Autodesk Inventor part; units mm, degrees
ref_plane "YZ Plane" through (0, 0, 0) normal (1, 0, 0) x (0, 1, 0)
ref_plane "XZ Plane" through (0, 0, 0) normal (0, 1, 0) x (-1, 0, 0)
ref_plane "XY Plane" through (0, 0, 0) normal (0, 0, 1) x (1, 0, 0)
sketch "Sketch1" plane through (0, 0, 0) normal (1, 0, 0) x (0, 1, 0)
  circle A0 centre (0, 0) radius 15.875
  circle A1 centre (18.7452, -32.4676) radius 4.0043
  circle A2 centre (18.7452, -32.4676) radius 15.875
  circle A3 centre (-37.4904, 0) radius 4.0043
  circle A4 centre (-37.4904, 0) radius 15.875
  circle A5 centre (18.7452, 32.4676) radius 15.875
  circle A6 centre (18.7452, 32.4676) radius 4.0043
  circle A7 centre (18.7452, -32.4676) radius 4.0043
  circle A8 centre (18.7452, -32.4676) radius 15.875
  circle A9 centre (0, 0) radius 15.875
  circle A10 centre (-37.4904, 0) radius 4.0043
  circle A11 centre (-37.4904, 0) radius 15.875
  circle A12 centre (18.7452, 32.4676) radius 4.0043
  circle A13 centre (18.7452, 32.4676) radius 15.875
  line L0 (34.6202, 32.4676) -> (34.6202, -32.4676)
  line L1 (10.8077, -46.2158) -> (-45.4279, -13.7482)
  line L2 (10.8077, 46.2158) -> (-45.4279, 13.7482)
  circle A14 centre (18.7452, 32.4676) radius 15.875
  circle A15 centre (-37.4904, 0) radius 15.875
  circle A16 centre (18.7452, -32.4676) radius 15.875
  circle A17 centre (41.995, 0) radius 14.4142
  circle A18 centre (-20.9975, 36.3687) radius 14.4142
  circle A19 centre (-20.9975, -36.3687) radius 14.4142
  point P0 (-28.0356, -23.7896)
  point P1 (-6.5846, -36.1743)
  point P2 (10.8077, -46.2158)
  point P3 (34.6202, -12.3847)
  point P4 (34.6202, 12.3847)
  point P5 (-6.5846, 36.1743)
  point P6 (-28.0356, 23.7896)
  point P7 (-45.4279, 13.7482)
  point P8 (-45.4279, -13.7482)
  dimension "d28" = 360
  dimension "d34" = 31.75
  dimension "d35" = 28.8284
  dimension "d36" = 8.0086
  dimension "d37" = 31.75
  dimension "d38" = 31.75
  dimension "d39" = 60
  dimension "d40" = 60
  dimension "d41" = 7.3748
  dimension "d42" = 55.6177
  dimension "d43" = 55.6177
  dimension "d44" = 0
  dimension "d45" = 41.2048
  dimension "d46" = 0
  dimension "d47" = 62.6558
  dimension "d48" = 80.0481
  dimension "d49" = 0
  dimension "d50" = 80.0481
  dimension "d51" = 15.875
  dimension "d52" = 15.875
  dimension "d53" = 23.8125
  dimension "d54" = 80.0481
  dimension "d55" = 34.6202
  dimension "d56" = 34.6202
  dimension "d57" = 41.2048
  dimension "d58" = 0
  dimension "d59" = 41.2048
  dimension "d60" = 62.6558
  dimension "d61" = 62.6558
  dimension "d62" = 0
  dimension "d63" = 62.6558
  dimension "d64" = 41.2048
  dimension "d65" = 72.1106
  dimension "d66" = 80.0481
  dimension "d67" = 0
  dimension "d68" = 80.0481
  dimension "d69" = 23.8125
extrude "Extrusion1" add sketch "Sketch1" along normal blind 8.255 contours A2 | A2 L1 A19 A4 L2 A18 A5 L0 A17 | A5 | A4
fillet "Fillet2" radius 3.175 6 edges at (4.1275, 34.6202, 12.3847) (4.1275, 34.6202, -12.3847) (4.1275, -6.5846, 36.1743) (4.1275, -28.0356, 23.7896) (4.1275, -6.5846, -36.1743) (4.1275, -28.0356, -23.7896)
sketch "Sketch5" plane through (8.255, 0, 0) normal (1, 0, 0) x (0, 0, -1)
  circle A0 centre (0, 0) radius 15.875
  circle A1 centre (0, 0) radius 12.7
  dimension "d70" = 25.4
extrude "Extrusion3" add sketch "Sketch5" against normal up to surface (8.255 mm away)
chamfer "Chamfer4" distance 0.254 angle 45 37 edges at (8.255, 2.8431, -41.6174) (8.255, 26.6827, -46.2158) (8.255, 34.6202, -23.2709) (8.255, 34.2848, -12.6539) (8.255, 27.5808, 0) (8.255, 34.2848, 12.6539) (8.255, 34.6202, 23.2709) (8.255, 26.6827, 46.2158) (8.255, 2.8431, 41.6174) (8.255, -6.1838, 36.0185) (8.255, -13.7904, 23.8857) (8.255, -28.101, 23.3646) (8.255, -37.4633, 18.3465) (8.255, -53.3654, 0) (8.255, -37.4633, -18.3465) (8.255, -28.101, -23.3646) (8.255, -13.7904, -23.8857) (8.255, -6.1838, -36.0185) (8.255, 0, 12.7) (0, 2.8431, 41.6174) (0, -6.1838, 36.0185) (0, -13.7904, 23.8857) (0, -28.101, 23.3646) (0, -37.4633, 18.3465) (0, -53.3654, 0) (0, -37.4633, -18.3465) (0, -28.101, -23.3646) (0, -13.7904, -23.8857) (0, -6.1838, -36.0185) (0, 2.8431, -41.6174) (0, 26.6827, -46.2158) (0, 34.6202, -23.2709) (0, 34.2848, -12.6539) (0, 27.5808, 0) (0, 34.2848, 12.6539) (0, 34.6202, 23.2709) (0, 26.6827, 46.2158)
properties part number "Torque_Triangle"
Design review of the part built by this model. Coordinates are the model's own, in mm. A direction names the side the tool comes from. Coordinates: 2 decimals unless noted, no trailing zeros. Loops run counter-clockwise (first coordinate to the right, second up) from the corner with the lowest first, then second, coordinate; pieces in that order, holes last.
Q1. We need section A-A on z = 0. State the section outline as (x, y) points (3 decimals).
Reported:
outline: (0, -53.111) - (0.254, -53.365) - (8.001, -53.365) - (8.255, -53.111) - (8.255, -41.495) - (0, -41.495) - close; (0, -33.486) - (8.255, -33.486) - (8.255, -12.954) - (8.001, -12.7) - (0, -12.7) - close; (0, 12.7) - (8.001, 12.7) - (8.255, 12.954) - (8.255, 27.327) - (8.001, 27.581) - (0.254, 27.581) - (0, 27.327) - close
Q2. The part is to be moulded in two halves that separate along Y. For faces 3 (the face through (4.07, -13.63, 23.98)), 4 (the face through (0.129, -37.289, 18.302)), 5 (the face through (8.255, -9, -10)), say which applies: +Y half, -Y half, draft (parallel to the pull), parting line (faces both ways), or undercut.
Reported:
face 3: undercut
face 4: -Y half
face 5: draft
Q3. We need section D-D on z = -16. State the section outline as (x, y) points (3 decimals).
Reported:
outline: (0, -41.02) - (0.254, -41.528) - (8.001, -41.528) - (8.255, -41.02) - (8.255, 34.366) - (8.001, 34.62) - (0.254, 34.62) - (0, 34.366) - close
Q4. We need section B-B on y = 0. State the section outline as (x, z) points (3 decimals).
Reported:
outline: (0, -39.683) - (0.254, -39.976) - (8.001, -39.976) - (8.255, -39.683) - (8.255, -12.954) - (8.001, -12.7) - (0, -12.7) - close; (0, 12.7) - (8.001, 12.7) - (8.255, 12.954) - (8.255, 39.683) - (8.001, 39.976) - (0.254, 39.976) - (0, 39.683) - close
Q5. We need section C-C on x = 5.75. State how many separate pieces and enclosed holes the cut face has, and give its area (3 significant figures).
Reported:
separate pieces: 1
enclosed holes: 4
area: 4,680 mm2
Q6. Tool access review of faces 1 (the face through (4.18, 34.28, 12.64)), 2 (the face through (4.182, -28.122, -23.363)): name each direction out of +Z, -Z, +X, -X, +Y, -Y from which nothing blocks a thin tool from reaching the whole face with its end or side.
Reported:
face 1: +X, -X, +Y
face 2: -Z, +X, -X
Q7. For pin 1 (13 mm diameter, centred on y = 18.75, z = -32.47, fed in from -X); pin 2 (1 mm diameter, centred on x = 6.5, z = 5.5, fed in from +Y); pin 3 (1 mm diameter, centred on x = 7, z = -3, fed in from +Y); pin 4 (1.5 mm diameter, centred on x = 3, y = -10, fed in from +Z), all flat-tipped, find the tip position at first contact; note any pin that passes through.
Reported:
pin 1: stops at x = 0
pin 2: stops at y = 28.89
pin 3: stops at y = 28.01
pin 4: stops at z = 28.02
Q8. To check wall thickness, follow line 1 (Y direction, x = 3, z = -2); line 2 (Z direction, x = 0.5, y = 15.5); line 3 (Y direction, x = 3, z = -3). State the ranges of each line that lie inside material, in increasing order.
Reported:
line 1: y = -53.24 to -40.96, -34.02 to -12.54, 12.54 to 27.72
line 2: z = -48.01 to -34.81, -30.12 to 30.12, 34.81 to 48.01
line 3: y = -53.08 to -40.14, -34.84 to -12.34, 12.34 to 27.9
